For this review, take the finished solid that the model builds, in its own axes (mm). Round coordinates to 2 decimals unless told otherwise and drop trailing zeros. Write each loop counter-clockwise with the first axis right and the second up, starting at its lowest first coordinate (ties: lowest second). Pieces come first, ordered by that corner, then holes. Notation, with made-up numbers: (35, 25.25) -> (62, 25.25) arc R22 ccw to (62, 44.25) -> close; hole circle Ø11 at (-0.5, 64). An arc over 180 degrees is marked (long way). Answer as CSV lines item,"result". Start each with the question number.
Item 1: Take a section at A-A on z = -228.6. Give the boundary of the cut face in (x, y), then the cut area to 3 significant figures.
Item 2: Wall thickness on probe 1 along Z at (x, y) = (4, 0) (3 decimals); probe 2 along Y at (x, z) = (-8.5, 190.5) (3 decimals); probe 3 along Y at (x, z) = (9, 190.5) (3 decimals): over which ranges is each line inside the solid? List them lowest first. Write a range as from..to.
Item 3: For pin 1 Ø3 at (x, z) = (-6, 9) entering from -Y; pin 2 Ø5.5 at (y, z) = (0, 241.3) entering from +X; pin 3 Ø8 at (y, z) = (6.5, 202.5) entering from -X; pin 4 Ø8 at (y, z) = (-8.5, 110.5) entering from +X, all flat-tipped, find the tip position at first contact; note any pin that passes through.
Item 4: Take a section at B-B on z = -29. Give the boundary of the cut face in (x, y).
```python
from build123d import *

# Parameters (mm, degrees)
SKETCH1_R               = 12.7
BOSS_EXTRUDE1_DEPTH     = 254
SKETCH2_R               = 3.175
SKETCH2_R_2             = 6.35
CUT_EXTRUDE1_DEPTH      = 13.7
CUT_EXTRUDE1_DEPTH_BACK = 13.7


with BuildPart() as part:
    # Sketch1 → Boss-Extrude1 (new body, symmetric)
    with BuildSketch(Plane.XY):
        Circle(SKETCH1_R)
    extrude(amount=BOSS_EXTRUDE1_DEPTH, both=True)

    # Sketch2 → Cut-Extrude1 (cut, two sides)
    with BuildSketch(Plane(origin=(0, 0, 0), x_dir=(0, 0, -1), z_dir=(1, 0, 0))) as cut_extrude1_sk:
        with Locations((-241.3, 0)):
            Circle(SKETCH2_R)
        with Locations((-190.5, 0)):
            Circle(SKETCH2_R)
        with Locations((228.6, 0)):
            Circle(SKETCH2_R_2)
    extrude(amount=CUT_EXTRUDE1_DEPTH, mode=Mode.SUBTRACT)
    extrude(cut_extrude1_sk.sketch, amount=-CUT_EXTRUDE1_DEPTH_BACK, mode=Mode.SUBTRACT)


solid = part.part
```
Output values:
1,outline,"(-11, -6.35) arc R12.7 ccw to (11, -6.35) -> close; (-11, 6.35) -> (11, 6.35) arc R12.7 ccw to start"
1,area,"198 mm^2"
2,probe 1,"z = -254..-234.95, -222.25..187.325, 193.675..238.125, 244.475..254"
2,probe 2,"y = -9.436..-3.175, 3.175..9.436"
2,probe 3,"y = -8.96..-3.175, 3.175..8.96"
3,pin 1,"stops at y = -11.88"
3,pin 2,"passes through"
3,pin 3,"stops at x = -12.45"
3,pin 4,"stops at x = 11.88"
4,outline,"circle Ø25.4 at (0, 0)"
